from build123d import *

# Parameters (mm, degrees)
F0_W     = 152.4
F0_H     = 254
F0_R     = 6.35
F1_DEPTH = 4.7625


with BuildPart() as f1:
    # F0 (on Right) → F1 (new body, symmetric)
    with BuildSketch(Plane.YZ):
        with Locations((-20.3339084785, 38.4282420009)):
            Rectangle(F0_W, F0_H)
        with Locations((5.0660915215, 114.6282420009)):
            Circle(F0_R, mode=Mode.SUBTRACT)
    extrude(amount=F1_DEPTH, both=True)


solid = f1.part
For this review, take the finished solid that the model builds, in its own axes (mm). Round coordinates to 2 decimals unless told otherwise and drop trailing zeros. Write each loop counter-clockwise with the first axis right and the second up, starting at its lowest first coordinate (ties: lowest second). Pieces come first, ordered by that corner, then holes. Notation, with made-up numbers: (40, 50) - (45, 50) arc R14 ccw to (45, 74) - close; hole circle Ø1 at (78.25, 65). An arc over 180 degrees is marked (long way). Use a Markdown table: item, result.
Q1. Wall thickness on line 1 along Y through (x, z) = (4.25, 113.5); line 2 along Z through (x, y) = (4, 6): over which ranges is each line inside the solid? List them lowest first.
Derived:
| item | result |
|---|---|
| line 1 | y = -96.53 to -1.18, 11.32 to 55.87 |
| line 2 | z = -88.57 to 108.35, 120.91 to 165.43 |
Q2. The part is to be moulded in two halves that separate along Y. For faces 1 (the cylindrical face through (-0.07, 3.69, 108.43)), 2 (the flat face through (4.762, -21, 40)), 3 (the flat face through (0, 55.866, 37)), say which applies: pulls with the +Y half, pulls with the -Y half, needs draft (parallel to the pull), parting line crosses it, or undercut.
Derived:
| item | result |
|---|---|
| face 1 | undercut |
| face 2 | needs draft |
| face 3 | pulls with the +Y half |
Q3. We need section A-A (y = 8.5). Give the boundary of the cut face in (x, z).
Derived:
| item | result |
|---|---|
| outline | (-4.76, -88.57) - (4.76, -88.57) - (4.76, 109.29) - (-4.76, 109.29) - close; (-4.76, 119.97) - (4.76, 119.97) - (4.76, 165.43) - (-4.76, 165.43) - close |
